```python
from build123d import *

# Parameters (mm, degrees)
SKETCH1_R           = 5
BOSS_EXTRUDE1_DEPTH = 8
FILLET1_R           = 4


with BuildPart() as part:
    # Sketch1 → Boss-Extrude1 (new body)
    with BuildSketch(Plane.XY):
        with BuildLine():
            Line((12.943190902, 5.109212861), (58.954715367, 9.945218954))
            ThreePointArc((58.954715367, 9.945218954), (70, 0), (58.954715367, -9.945218954))
            Line((58.954715367, -9.945218954), (12.943190902, -5.109212861))
            ThreePointArc((12.943190902, -5.109212861), (11.32982846, -5.388970193), (10.103684409, -6.474222838))
            ThreePointArc((10.103684409, -6.474222838), (0, -12), (-10.103684409, -6.474222838))
            ThreePointArc((-10.103684409, -6.474222838), (-11.32982846, -5.388970193), (-12.943190902, -5.109212861))
            Line((-12.943190902, -5.109212861), (-58.954715367, -9.945218954))
            ThreePointArc((-58.954715367, -9.945218954), (-70, 0), (-58.954715367, 9.945218954))
            Line((-58.954715367, 9.945218954), (-12.943190902, 5.109212861))
            ThreePointArc((-12.943190902, 5.109212861), (-11.32982846, 5.388970193), (-10.103684409, 6.474222838))
            ThreePointArc((-10.103684409, 6.474222838), (0, 12), (10.103684409, 6.474222838))
            ThreePointArc((10.103684409, 6.474222838), (11.32982846, 5.388970193), (12.943190902, 5.109212861))
        make_face()
        Circle(SKETCH1_R, mode=Mode.SUBTRACT)
    extrude(amount=BOSS_EXTRUDE1_DEPTH)

    # Fillet1
    fillet1_edges = [part.edges().sort_by_distance(p)[0] for p in [
        (0, 12, 0),
        (-11.32982846, -5.388970193, 0),
        (70, 0, 8),
        (-35.948953134, -7.527215907, 0),
        (-70, 0, 0),
        (-35.948953134, 7.527215907, 0),
        (-11.32982846, 5.388970193, 0),
        (11.32982846, 5.388970193, 0),
        (35.948953134, 7.527215907, 0),
        (35.948953134, -7.527215907, 0),
        (11.32982846, -5.388970193, 0),
        (35.948953134, 7.527215907, 8),
        (-35.948953134, 7.527215907, 8),
        (-35.948953134, -7.527215907, 8),
        (35.948953134, -7.527215907, 8),
    ]]
    fillet(fillet1_edges, radius=FILLET1_R - 0.0001)  # a hair under: the kernel refuses the full size


solid = part.part
```
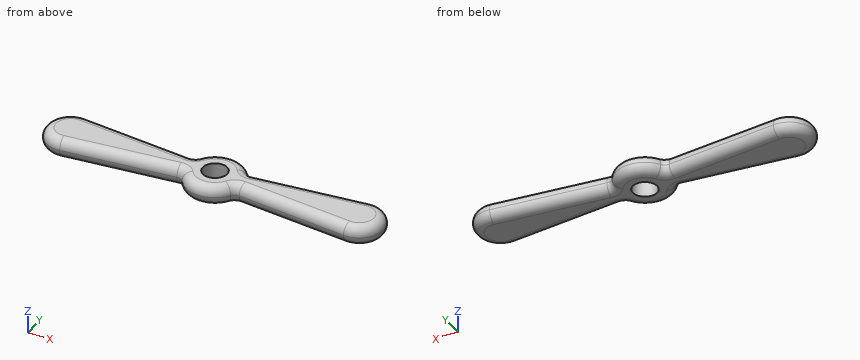
Read the model definition and answer for the solid it produces. Units are mm, in the model's axes. Coordinates: 2 decimals unless noted, no trailing zeros. Write each loop counter-clockwise with the first axis right and the second up, starting at its lowest first coordinate (ties: lowest second). Pieces come first, ordered by that corner, then holes. Notation, with made-up numbers: (41, 77) - (92, 77) arc R16 cw to (92, 96) - close; hole circle Ø7 at (-4, 20). An arc over 180 degrees is marked (long way). Answer as a JSON object with one key per item and string values. Group by question number.
1. A cutting plane is placed at B-B (z = 2). Determine the outline of the cut face in (x, y).
2. Each of these flat-tipped pins is pushed along its axis until it touches: P1, Ø3, axis at x = 16, z = 3, coming from the +Y side; P2, Ø1, axis at x = -15, y = -2, coming from the +Z side. Where does it stop, or does it pass through?
3. Consider L1, parallel to Z at x = -43, y = -4.5; L2, parallel to Y at x = 0, z = 2.25; L3, parallel to X at y = -3.5, z = 4.75. Determine where each line is inside the solid, lowest interval first. Write a range as [from, to].
Worked out:
{
 "1": {"outline": "(-59.01, -9.41) - (-13, -4.58) arc R3.54 cw to (-9.65, -6.19) arc R11.46 ccw to (9.65, -6.19) arc R3.54 cw to (13, -4.58) - (59.01, -9.41) arc R9.46 ccw (long way) to (59.01, 9.41) - (13, 4.58) arc R3.54 cw to (9.65, 6.19) arc R11.46 ccw to (-9.65, 6.19) arc R3.54 cw to (-13, 4.58) - (-59.01, 9.41) arc R9.46 ccw (long way) to start; hole circle Ø10 at (0, 0)"},
 "2": {"P1": "stops at y = 5.56", "P2": "stops at z = 8"},
 "3": {"L1": "z = [0.01, 7.99]", "L2": "y = [-11.6, -5], [5, 11.6]", "L3": "x = [-69.29, -3.57], [3.57, 69.29]"}
}
